Build history of the part. All positions in model axes, mm. Face numbers are marked on the shaded views. A direction names the side the tool comes from. Coordinates: 2 decimals unless noted, no trailing zeros. Loops run counter-clockwise (first coordinate to the right, second up) from the corner with the lowest first, then second, coordinate; pieces in that order, holes last.
(1) Slice it at C-C (z = 17). Give the cut face in (x, y).
(2) Slice it at B-B (y = 5). Give the cut face in (x, z), and give its area (3 significant figures).
(3) Tool access for the marked faces 1, 2 and 3: list every direction of +Z, -Z, +X, -X, +Y, -Y with a clear straight run to the whole face (end or side of a thin tool).
(4) Slice it at A-A (x = 0). Give the cut face in (y, z), and give its area (4 significant figures).
(5) Wall check: L1, parallel to Z at x = -4.5, y = 2.75; L2, parallel to Y at x = 0.25, z = 21.5; L3, parallel to X at y = 5.5, z = 17. Give the ranges that are in metal, low to high.
(6) Flat gauge pins, fed straight in: P1, Ø3, axis at y = 7, z = 19.5, coming from the -X side; P2, Ø2, axis at x = 0.5, y = 7.5, coming from the +Z side; P3, Ø0.7, axis at x = 0, z = 20.5, coming from the +Y side. Where does each tip first touch, or does it go through?
(7) Slice it at D-D (y = 7.5). Give the cut face in (x, z), and give its area (3 significant figures).
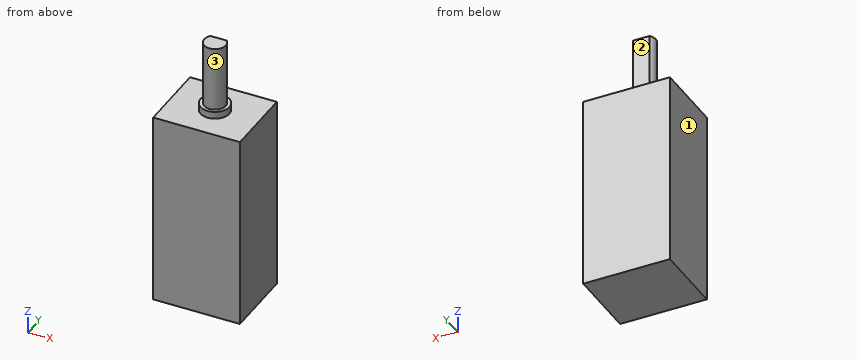
from build123d import *

# Parameters (mm, degrees)
SKETCH2_W           = 12
SKETCH2_H           = 27
BOSS_EXTRUDE1_DEPTH = 10
SKETCH4_R           = 2
BOSS_EXTRUDE2_DEPTH = 1
BOSS_EXTRUDE3_DEPTH = 9


with BuildPart() as part:
    # Sketch2 → Boss-Extrude1 (new body)
    with BuildSketch(Plane(origin=(0, 0, 0), x_dir=(1, 0, 0), z_dir=(0, 1, 0))):
        Rectangle(SKETCH2_W, SKETCH2_H)
    extrude(amount=BOSS_EXTRUDE1_DEPTH)

    # Sketch4 → Boss-Extrude2 (add)
    with BuildSketch(Plane.XY.offset(13.5)):
        with Locations((0, 5)):
            Circle(SKETCH4_R)
    extrude(amount=BOSS_EXTRUDE2_DEPTH)

    # Sketch5 → Boss-Extrude3 (add)
    with BuildSketch(Plane.XY.offset(14.5)):
        with BuildLine():
            Line((-1.118033989, 6), (1.118033989, 6))
            ThreePointArc((1.118033989, 6), (0, 3.5), (-1.118033989, 6))
        make_face()
    extrude(amount=BOSS_EXTRUDE3_DEPTH)


solid = part.part
Response values:
1. outline: (-1.12, 6) arc R1.5 ccw (long way) to (1.12, 6) - close
2. outline: (-6, -13.5) - (6, -13.5) - (6, 13.5) - (2, 13.5) - (2, 14.5) - (1.5, 14.5) - (1.5, 23.5) - (-1.5, 23.5) - (-1.5, 14.5) - (-2, 14.5) - (-2, 13.5) - (-6, 13.5) - close
2. area: 355 mm2
3. face 1: +Z, -Z, -X, +Y, -Y
3. face 2: +Z, +X, -X, +Y
3. face 3: +Z
4. outline: (0, -13.5) - (10, -13.5) - (10, 13.5) - (7, 13.5) - (7, 14.5) - (6, 14.5) - (6, 23.5) - (3.5, 23.5) - (3.5, 14.5) - (3, 14.5) - (3, 13.5) - (0, 13.5) - close
4. area: 296.5 mm2
5. L1: z = -13.5 to 13.5
5. L2: y = 3.52 to 6
5. L3: x = -1.41 to 1.41
6. P1: stops at x = -1.41
6. P2: stops at z = 14.5
6. P3: stops at y = 6
7. outline: (-6, -13.5) - (6, -13.5) - (6, 13.5) - (-6, 13.5) - close
7. area: 324 mm2
